The model under review builds one solid part; all positions refer to its coordinate system, in mm. Round coordinates to 2 decimals unless told otherwise and drop trailing zeros. Write each loop counter-clockwise with the first axis right and the second up, starting at its lowest first coordinate (ties: lowest second). Pieces come first, ordered by that corner, then holes.
Item 1: Clearance check with flat-ended pins moving along their axes: pin 1 Ø1.6 at (x, y) = (-79.5, 35) entering from -Z; pin 2 Ø8 at (x, z) = (-80.5, 130) entering from -Y (3 decimals); pin 3 Ø1 at (x, y) = (-54, 35) entering from +Z; pin 4 Ø1 at (x, y) = (-78.5, 34) entering from +Z. State where each tip first meets the part, or that it passes through.
Item 2: Add section C-C (y = 33.9). State how many separate pieces and enclosed holes the cut face has, plus the area to 3 significant figures.
Item 3: Add section B-B (z = 98.6). Give the boundary of the cut face in (x, y) (3 decimals).
Item 4: Add section A-A (z = 113.5). Give the boundary of the cut face in (x, y) (3 decimals).
Item 5: Add section D-D (x = -69). Give the boundary of the cut face in (y, z) (3 decimals), plus the area to 3 significant figures.
Item 6: To check wall thickness, follow L1, parallel to X at y = 33.2, z = 116; L2, parallel to Z at x = -77.5, y = 34.8; L3, parallel to Z at x = -84, y = 35.05. State the ranges of each line that lie inside material, in increasing order.
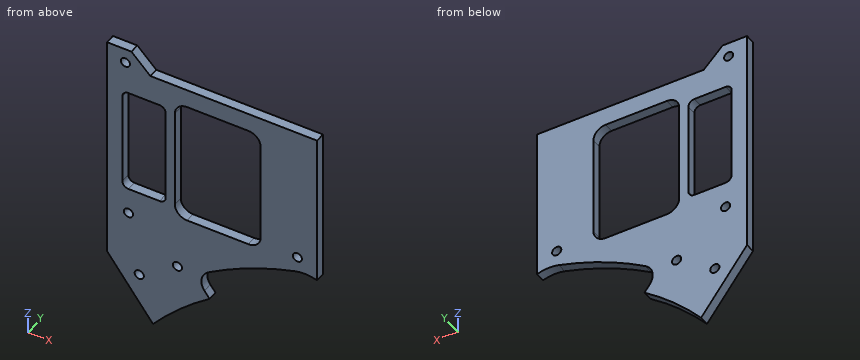
```python
from build123d import *

# Parameters (mm, degrees)
SKETCH1_R                    = 7
SKETCH1_R_2                  = 3.9
SKETCH1_R_3                  = 1.3
SKETCH1_W                    = 14.16
SKETCH1_H                    = 34.693281024
BOSS_EXTRUDE1_DEPTH          = 3.175
FILLET1_R                    = 2
SKETCH2_R                    = 1.5
CUT_EXTRUDE1_DEPTH           = 4.175
SKETCH5_W                    = 28
SKETCH5_H                    = 41
CUT_EXTRUDE3_DEPTH           = 4.175
FILLET2_R                    = 4
SKETCH10_R                   = 1.5
NOSE_GUARD_SCREW_HOLES_DEPTH = 4.175
SKETCH11_R                   = 20
CUT_EXTRUDE4_DEPTH           = 4.175
SKETCH12_R                   = 1.5
CUT_EXTRUDE5_DEPTH           = 4.175
SKETCH13_R                   = 96.550525729
CUT_EXTRUDE6_DEPTH           = 4.175
SKETCH14_W                   = 292.522671741
SKETCH14_H                   = 256.088396318
CUT_EXTRUDE7_DEPTH           = 4.175


with BuildPart() as part:
    # Sketch1 → Boss-Extrude1 (new body)
    with BuildSketch(Plane(origin=(0, 32.825, 0), x_dir=(1, 0, 0), z_dir=(0, 1, 0))):
        with BuildLine():
            Line((89.16, -81.763233191), (17.569981221, 13.239930509))
            ThreePointArc((17.569981221, 13.239930509), (0, 22), (-17.569981221, 13.239930509))
            Line((-17.569981221, 13.239930509), (-89.16, -81.763233191))
            Line((-89.16, -81.763233191), (-89.16, -157.357359313))
            Line((-89.16, -157.357359313), (-81.189437252, -157.357359313))
            Line((-81.189437252, -157.357359313), (-75.032077939, -151.2))
            Line((-75.032077939, -151.2), (75.032077939, -151.2))
            Line((75.032077939, -151.2), (81.189437252, -157.357359313))
            Line((81.189437252, -157.357359313), (89.16, -157.357359313))
            Line((89.16, -157.357359313), (89.16, -81.763233191))
        make_face()
        with Locations((0, -124.6)):
            Circle(SKETCH1_R, mode=Mode.SUBTRACT)
        Circle(SKETCH1_R_2, mode=Mode.SUBTRACT)
        with Locations((0, -28)):
            Circle(SKETCH1_R_3, mode=Mode.SUBTRACT)
        with Locations((-77.08, -124.6)):
            Rectangle(SKETCH1_W, SKETCH1_H, mode=Mode.SUBTRACT)
        with Locations((77.08, -124.6)):
            Rectangle(SKETCH1_W, SKETCH1_H, mode=Mode.SUBTRACT)
        with BuildLine():
            Line((-21.49317755, -33.507330392), (-57.351202685, -81.09253696))
            ThreePointArc((-57.351202685, -81.09253696), (-58.277395442, -84.995925096), (-56.036640854, -88.323580553))
            ThreePointArc((-56.036640854, -88.323580553), (-42.323470644, -95.65502513), (-27.674946004, -100.872480705))
            ThreePointArc((-27.674946004, -100.872480705), (-17.223302674, -98.842107372), (-12.5, -89.300111982))
            Line((-12.5, -89.300111982), (-12.5, -36.516405507))
            ThreePointArc((-12.5, -36.516405507), (-15.913476718, -31.774787231), (-21.49317755, -33.507330392))
        make_face(mode=Mode.SUBTRACT)
        with BuildLine():
            Line((57.351202685, -81.09253696), (21.49317755, -33.507330392))
            ThreePointArc((21.49317755, -33.507330392), (15.913476718, -31.774787231), (12.5, -36.516405507))
            Line((12.5, -36.516405507), (12.5, -89.300111982))
            ThreePointArc((12.5, -89.300111982), (17.223302674, -98.842107372), (27.674946004, -100.872480705))
            ThreePointArc((27.674946004, -100.872480705), (42.323470644, -95.65502513), (56.036640854, -88.323580553))
            ThreePointArc((56.036640854, -88.323580553), (58.277395442, -84.995925096), (57.351202685, -81.09253696))
        make_face(mode=Mode.SUBTRACT)
    extrude(amount=BOSS_EXTRUDE1_DEPTH)

    # Fillet1
    fillet1_edges = [part.edges().sort_by_distance(p)[0] for p in [
        (-84.16, 34.4125, 107.253359488),
        (-84.16, 34.4125, 141.946640512),
        (-70, 34.4125, 141.946640512),
        (-70, 34.4125, 107.253359488),
        (84.16, 34.4125, 107.253359488),
        (70, 34.4125, 107.253359488),
        (70, 34.4125, 141.946640512),
        (84.16, 34.4125, 141.946640512),
    ]]
    fillet(fillet1_edges, radius=FILLET1_R)

    # Sketch2 → Cut-Extrude1 (cut, through all)
    with BuildSketch(Plane(origin=(0, 36, 0), x_dir=(1, 0, 0), z_dir=(0, 1, 0))):
        with Locations((-62.088932188, -184.6)):
            Circle(SKETCH2_R)
        with Locations((-27, -106.222219898)):
            Circle(SKETCH2_R)
        with Locations((-83.16, -152.6)):
            Circle(SKETCH2_R)
        with Locations((-78.638732223, -77.770880118)):
            Circle(SKETCH2_R)
        with Locations((27, -106.222219898)):
            Circle(SKETCH2_R)
        with Locations((62.088932188, -184.6)):
            Circle(SKETCH2_R)
        with Locations((83.16, -162.114718626)):
            Circle(SKETCH2_R)
        with Locations((78.638732223, -77.770880118)):
            Circle(SKETCH2_R)
        with Locations((83.16, -152.6)):
            Circle(SKETCH2_R)
        with Locations((-83.16, -162.114718626)):
            Circle(SKETCH2_R)
    extrude(amount=-CUT_EXTRUDE1_DEPTH, mode=Mode.SUBTRACT)

    # Sketch5 → Cut-Extrude3 (cut, through all)
    with BuildSketch(Plane(origin=(0, 36, 0), x_dir=(1, 0, 0), z_dir=(0, 1, 0))):
        with Locations((-53, -124.6)):
            Rectangle(SKETCH5_W, SKETCH5_H)
        with Locations((53, -124.6)):
            Rectangle(SKETCH5_W, SKETCH5_H)
    extrude(amount=-CUT_EXTRUDE3_DEPTH, mode=Mode.SUBTRACT)

    # Fillet2
    fillet2_edges = [part.edges().sort_by_distance(p)[0] for p in [
        (-67, 34.4125, 145.1),
        (-67, 34.4125, 104.1),
        (-39, 34.4125, 104.1),
        (-39, 34.4125, 145.1),
        (67, 34.4125, 104.1),
        (67, 34.4125, 145.1),
        (39, 34.4125, 145.1),
        (39, 34.4125, 104.1),
    ]]
    fillet(fillet2_edges, radius=FILLET2_R)

    # Sketch10 → nose-guard-screw-holes (cut, through all)
    with BuildSketch(Plane(origin=(0, 36, 0), x_dir=(1, 0, 0), z_dir=(0, 1, 0))):
        with Locations((0, 17)):
            Circle(SKETCH10_R)
        with Locations((-14.722431864, 8.5)):
            Circle(SKETCH10_R)
        with Locations((14.722431864, 8.5)):
            Circle(SKETCH10_R)
        with Locations((0, -44.25832974)):
            Circle(SKETCH10_R)
        with Locations((0, -67.77856843)):
            Circle(SKETCH10_R)
        with Locations((0, -91.29880712)):
            Circle(SKETCH10_R)
    extrude(amount=-NOSE_GUARD_SCREW_HOLES_DEPTH, mode=Mode.SUBTRACT)

    # Sketch11 → Cut-Extrude4 (cut, through all)
    with BuildSketch(Plane(origin=(0, 36, 0), x_dir=(1, 0, 0), z_dir=(0, 1, 0))):
        with Locations((0, -124.6)):
            Circle(SKETCH11_R)
    extrude(amount=-CUT_EXTRUDE4_DEPTH, mode=Mode.SUBTRACT)

    # Sketch12 → Cut-Extrude5 (cut, through all)
    with BuildSketch(Plane(origin=(0, 36, 0), x_dir=(1, 0, 0), z_dir=(0, 1, 0))):
        with Locations((-82.16, -98.6)):
            Circle(SKETCH12_R)
        with Locations((66.171704332, -86.11193614)):
            Circle(SKETCH12_R)
        with Locations((82.16, -98.6)):
            Circle(SKETCH12_R)
        with Locations((-66.171704332, -86.11193614)):
            Circle(SKETCH12_R)
    extrude(amount=-CUT_EXTRUDE5_DEPTH, mode=Mode.SUBTRACT)

    # Sketch13 → Cut-Extrude6 (cut, through all)
    with BuildSketch(Plane(origin=(0, 36, 0), x_dir=(1, 0, 0), z_dir=(0, 1, 0))):
        Circle(SKETCH13_R)
    extrude(amount=-CUT_EXTRUDE6_DEPTH, mode=Mode.SUBTRACT)

    # Sketch14 → Cut-Extrude7 (cut, through all)
    with BuildSketch(Plane(origin=(0, 36, 0), x_dir=(1, 0, 0), z_dir=(0, 1, 0))):
        with Locations((125.685144355, -44.004038114)):
            Rectangle(SKETCH14_W, SKETCH14_H)
    extrude(amount=-CUT_EXTRUDE7_DEPTH, mode=Mode.SUBTRACT)


solid = part.part
```
Numbers:
1. pin 1: stops at z = 67.88
1. pin 2: stops at y = 32.825
1. pin 3: stops at z = 151.2
1. pin 4: stops at z = 155.17
2. separate pieces: 1
2. enclosed holes: 7
2. area: 2,980 mm2
3. outline: (-89.16, 32.825) - (-83.66, 32.825) - (-83.66, 36) - (-89.16, 36) - close; (-80.66, 32.825) - (-34.917, 32.825) - (-34.917, 36) - (-80.66, 36) - close
4. outline: (-89.16, 32.825) - (-84.16, 32.825) - (-84.16, 36) - (-89.16, 36) - close; (-70, 32.825) - (-67, 32.825) - (-67, 36) - (-70, 36) - close; (-39, 32.825) - (-20.576, 32.825) - (-20.576, 36) - (-39, 36) - close
5. outline: (32.825, 67.535) - (36, 67.535) - (36, 151.2) - (32.825, 151.2) - close
5. area: 266 mm2
6. L1: x = -89.16 to -84.16, -70 to -67, -39 to -20.58
6. L2: z = 66.29 to 76.79, 78.75 to 107.25, 141.95 to 153.67
6. L3: z = 74.92 to 108.47, 140.73 to 151.36, 153.84 to 157.36
